Read the model definition and answer for the solid it produces. Units are mm, in the model's axes. A direction names the side the tool comes from. Coordinates: 2 decimals unless noted, no trailing zeros. Write each loop counter-clockwise with the first axis right and the second up, starting at its lowest first coordinate (ties: lowest second). Pieces come first, ordered by that corner, then holes. Notation, with made-up numbers: (-10.5, 38) -> (3.5, 38) arc R24 ccw to (3.5, 71) -> close; hole circle Ø11 at (65.5, 2.5). An arc over 180 degrees is marked (long way). Write item = value, one per line. Start each with the question number.
1) For a pull along Z with two mould halves and no side action, classify faces 1 (the face through (-0.45, -3.85, 1.43)), 2 (the face through (0, -8, 0)), 3 (the face through (0, 0.5, 0)) as released by +Z, released by -Z, zero draft, split by the parting line, or undercut.
2) Section A-A (x = 0) is taken. Determine the outline of the cut face in (y, z), plus the area to 3 significant figures.
3) Flat-ended cylindrical pins translate along their axes: pin 1 Ø1.5 at (y, z) = (-5, 1.5) entering from -X; pin 2 Ø1.5 at (x, y) = (2.5, -5) entering from -Z; pin 3 Ø3 at (x, y) = (0.5, -5.5) entering from +Z; pin 4 Ø1.5 at (y, z) = (-5, -1) entering from +X. Find the tip coordinate at first contact, or state that the pin passes through.
4) A tool of negligible diameter and unlimited length cuts with its end or side. For faces 4 (the face through (-1.434, 2.848, 0.811)), 5 (the face through (-1.3, 0, 1.3)), 6 (the face through (0.9, 1.33, 2.86)), from which of +Z, -Z, +X, -X, +Y, -Y can it reach the whole face along a straight path? Write none if from no direction.
5) Find the intervals of material crossed by line 1 along X through (y, z) = (1.5, 2.4); line 2 along Z through (x, y) = (-0.05, -4.75); line 3 along X through (y, z) = (0.75, -1.1), in increasing order. Write a range as from..to.
6) Section B-B (y = -7) is taken. Determine the outline of the cut face in (x, z).
from build123d import *

# Parameters (mm, degrees)
SKETCH1_R           = 3
BOSS_EXTRUDE1_DEPTH = 3
CHAMFER1_SIZE       = 0.3
CUT_EXTRUDE1_DEPTH  = 2.5
CHAMFER2_SIZE       = 0.3
SKETCH3_R           = 1.5
BOSS_EXTRUDE2_DEPTH = 8
CHAMFER3_SIZE       = 0.2


with BuildPart() as part:
    # Sketch1 → Boss-Extrude1 (new body)
    with BuildSketch(Plane(origin=(0, 0, 0), x_dir=(1, 0, 0), z_dir=(0, 1, 0))):
        with Locations(Location((0, 0, 0), (0, 0, 270))):  # turned: the seam where the file's is
            Circle(SKETCH1_R)
    extrude(amount=BOSS_EXTRUDE1_DEPTH)

    # Chamfer1
    chamfer1_edges = [part.edges().sort_by_distance(p)[0] for p in [
        (0, 3, -3),
    ]]
    chamfer(chamfer1_edges, length=CHAMFER1_SIZE)

    # Sketch2 → Cut-Extrude1 (cut)
    with BuildSketch(Plane(origin=(0, 3, 0), x_dir=(1, 0, 0), z_dir=(0, 1, 0))):
        Polygon((1.732050808, 0), (0.866025404, 1.5), (-0.866025404, 1.5), (-1.732050808, 0), (-0.866025404, -1.5), (0.866025404, -1.5), align=None)
    extrude(amount=-CUT_EXTRUDE1_DEPTH, mode=Mode.SUBTRACT)

    # Chamfer2
    chamfer2_edges = [part.edges().sort_by_distance(p)[0] for p in [
        (1.299038106, 3, 0.75),
        (1.299038106, 3, -0.75),
        (0, 3, -1.5),
        (-1.299038106, 3, -0.75),
        (-1.299038106, 3, 0.75),
        (0, 3, 1.5),
    ]]
    chamfer(chamfer2_edges, length=CHAMFER2_SIZE)

    # Sketch3 → Boss-Extrude2 (add)
    with BuildSketch(Plane.XZ):
        with Locations(Location((0, 0, 0), (0, 0, 90))):  # turned: the seam where the file's is
            Circle(SKETCH3_R)
    extrude(amount=BOSS_EXTRUDE2_DEPTH)

    # Chamfer3
    chamfer3_edges = [part.edges().sort_by_distance(p)[0] for p in [
        (0, -8, -1.5),
    ]]
    chamfer(chamfer3_edges, length=CHAMFER3_SIZE)


solid = part.part
Answer key:
q1.face_1 = split by the parting line
q1.face_2 = zero draft
q1.face_3 = undercut
q2.outline = (-8, -1.3) -> (-7.8, -1.5) -> (0, -1.5) -> (0, -3) -> (2.7, -3) -> (3, -2.7) -> (3, -1.8) -> (2.7, -1.5) -> (0.5, -1.5) -> (0.5, 1.5) -> (2.7, 1.5) -> (3, 1.8) -> (3, 2.7) -> (2.7, 3) -> (0, 3) -> (0, 1.5) -> (-7.8, 1.5) -> (-8, 1.3) -> close
q2.area = 34.3 mm^2
q3.pin_1 = -1.3
q3.pin_2 = through
q3.pin_3 = 1.5
q3.pin_4 = 1.48
q4.face_4 = +Y
q4.face_5 = -Y
q4.face_6 = +Y, -Y
q5.line_1 = -1.8..1.8
q5.line_2 = -1.5..1.5
q5.line_3 = -2.79..-1.1, 1.1..2.79
q6.outline = circle Ø3 at (0, 0)
